from build123d import *

# Parameters (mm, degrees)
F1_DEPTH     = 2
F2_R         = 2
F3_R         = 2
F4_T4_DEPTH  = 22.7509646446
F4_T9_DEPTH  = 22.7509646446
F4_T14_DEPTH = 22.7509646446
F5_T4_DEPTH  = 22.7509646446
F5_T9_DEPTH  = 22.7509646446
F6_T4_DEPTH  = 22.7509646446


# Not quite as in the source:
# - a fillet or chamfer that OpenCascade refuses, or shapes differently, is made with other operations: its cross-section is extruded or revolved along the edge and cut away or added


with BuildPart() as f1:
    # F0 (on Top) → F1 (new body)
    with BuildSketch(Plane.XY):
        Polygon((-8.2, 10.65), (-14.2, 10.65), (-14.2, 0), (-8.2, -14.45), (-3.2, -14.45), (-3.2, -10.45), (-6.2, -10.45), (-6.2, -9.45), (-3.2, -9.45), (-3.2, -5.95), (-8.2, -5.95), (-8.2, 1), (-11.2, 1), (-11.2, 2), (-8.2, 2), (-8.2, 5.65), (-11.2, 5.65), (-11.2, 6.65), (-8.2, 6.65), align=None)
    extrude(amount=F1_DEPTH)

    # F2
    f2_edges = [f1.edges().sort_by_distance(p)[0] for p in [
        (-14.2, 10.65, 1),
        (-14.2, 0, 1),
        (-8.2, 10.65, 1),
        (-8.2, -14.45, 1),
        (-3.2, -14.45, 1),
        (-3.2, -5.95, 1),
    ]]
    fillet(f2_edges, radius=F2_R)

    # F3
    f3_edges = [f1.edges().sort_by_distance(p)[0] for p in [
        (-8.2, -5.95, 1),
    ]]
    fillet(f3_edges, radius=F3_R)

    # F4: chamfer of 1.5 x 4 on 3 edges, made by hand


with BuildPart() as f4_tool2:
    # F4_s3 → F4_t4 (new body)
    with BuildSketch(Plane.XY.offset(-10.3754823223)):
        Polygon((-12.2, 6.65), (-8.2, 8.15), (-8.2, 6.65), align=None)
    extrude(amount=F4_T4_DEPTH)

    split(bisect_by=Plane.YZ.offset(-11.2), keep=Keep.TOP)


with BuildPart() as f1_1:
    add(f1.part)

    # F4_t1: cut F4_tool2
    add(f4_tool2.part, mode=Mode.SUBTRACT)


with BuildPart() as f4_tool7:
    # F4_s8 → F4_t9 (new body)
    with BuildSketch(Plane.XY.offset(-10.3754823223)):
        Polygon((-12.2, 2), (-8.2, 3.5), (-8.2, 2), align=None)
    extrude(amount=F4_T9_DEPTH)

    split(bisect_by=Plane.YZ.offset(-11.2), keep=Keep.TOP)


with BuildPart() as f1_2:
    add(f1_1.part)

    # F4_t6: cut F4_tool7
    add(f4_tool7.part, mode=Mode.SUBTRACT)


with BuildPart() as f4_tool12:
    # F4_s13 → F4_t14 (new body)
    with BuildSketch(Plane.XY.offset(-10.3754823223)):
        Polygon((-3.2, -7.95), (-7.2, -9.45), (-3.2, -9.45), align=None)
    extrude(amount=F4_T14_DEPTH)

    split(bisect_by=Plane.YZ.offset(-6.2), keep=Keep.TOP)


with BuildPart() as f1_3:
    add(f1_2.part)

    # F4_t11: cut F4_tool12
    add(f4_tool12.part, mode=Mode.SUBTRACT)

    # F5: chamfer of 4 x 1.5 on 2 edges, made by hand


with BuildPart() as f5_tool2:
    # F5_s3 → F5_t4 (new body)
    with BuildSketch(Plane.XY.offset(-10.3754823223)):
        Polygon((-12.2, 5.65), (-8.2, 4.15), (-8.2, 5.65), align=None)
    extrude(amount=F5_T4_DEPTH)

    split(bisect_by=Plane.YZ.offset(-11.2), keep=Keep.TOP)


with BuildPart() as f1_4:
    add(f1_3.part)

    # F5_t1: cut F5_tool2
    add(f5_tool2.part, mode=Mode.SUBTRACT)


with BuildPart() as f5_tool7:
    # F5_s8 → F5_t9 (new body)
    with BuildSketch(Plane.XY.offset(-10.3754823223)):
        Polygon((-7.2, -10.45), (-3.2, -11.95), (-3.2, -10.45), align=None)
    extrude(amount=F5_T9_DEPTH)

    split(bisect_by=Plane.YZ.offset(-6.2), keep=Keep.TOP)


with BuildPart() as f1_5:
    add(f1_4.part)

    # F5_t6: cut F5_tool7
    add(f5_tool7.part, mode=Mode.SUBTRACT)

    # F6: chamfer of 4 x 1.5 on 1 edges, made by hand


with BuildPart() as f6_tool2:
    # F6_s3 → F6_t4 (new body)
    with BuildSketch(Plane.XY.offset(-10.3754823223)):
        Polygon((-12.2, 1), (-8.2, -0.5), (-8.2, 1), align=None)
    extrude(amount=F6_T4_DEPTH)

    split(bisect_by=Plane.YZ.offset(-11.2), keep=Keep.TOP)


with BuildPart() as f1_6:
    add(f1_5.part)

    # F6_t1: cut F6_tool2
    add(f6_tool2.part, mode=Mode.SUBTRACT)


solid = f1_6.part
Geometry: final body of the model. Coordinates: model frame, mm. A direction names the side the tool comes from. Coordinates: 2 decimals unless noted, no trailing zeros. Loops run counter-clockwise (first coordinate to the right, second up) from the corner with the lowest first, then second, coordinate; pieces in that order, holes last. Notation, with made-up numbers: (45.5, 75.5) - (70.5, 75.5) arc R21 cw to (70.5, 94.5) - close; hole circle Ø4 at (-37, 10.5). An arc over 180 degrees is marked (long way). Put each result on its own line as item: value. Start each with the question number.
Q1. Line query: line 1 (Y direction, x = -10.25, z = 1.75); line 2 (Y direction, x = -9, z = 1.45); line 3 (X direction, y = 8.5, z = 1.2). Output: solid intervals per line, ascending.
Q2. Cut plane C-C, the plane x = -3.75. Return loops of the section in (y, z).
Q3. Pin query (flat end, axial travel): pin 1 Ø1 at (y, z) = (-2.5, 0.5) entering from +X; pin 2 Ø0.9 at (y, z) = (6.5, 1.5) entering from +X; pin 3 Ø1.1 at (x, z) = (-5.5, 1) entering from +Y. Return the tip coordinate at first contact, or that it passes through.
Q4. Cut plane D-D, the plane y = 4.75. Return loops of the section in (x, z).
Q5. Set-up query: faces 5 (the cylindrical face through (-3.8, -13.88, 1.01)), 6 (the flat face through (-4.679, -8.505, 0.986)), 7 (the flat face through (-6, -5.95, 1)). Return all of +Z, -Z, +X, -X, +Y, -Y with unobstructed straight access to the full face (end or side cutting, diameter ignored); none if empty.
Q6. Cut plane B-B, the plane x = -9.75. Return loops of the section in (y, z).
Q7. Pull-direction query (Y, two-part tool) for faces 1 (the flat face through (-10, -2, 0)), 2 (the flat face through (-9.72, 0.07, 0.99)), 3 (the cylindrical face through (-13.6, 10.08, 1.01)), 4 (the cylindrical face through (-7.989, -14.104, 1.014)); classes: released by +Y, released by -Y, zero draft, split by the parting line, or undercut.
Q8. Cut plane A-A, the plane z = 0.5. Return loops of the section in (x, y) (3 decimals), and give its area (3 significant figures).
Filled sheet:
1. line 1: -9.51 to 0.27, 2.73 to 4.92, 7.38 to 10.65
1. line 2: -12.52 to -0.2, 3.2 to 4.45, 7.85 to 10.25
1. line 3: -14.2 to -8.2
2. outline: (-13.83, 0) - (-11.74, 0) - (-11.74, 2) - (-13.83, 2) - close; (-8.16, 0) - (-6.57, 0) - (-6.57, 2) - (-8.16, 2) - close
3. pin 1: x = -8.2
3. pin 2: x = -11.2
3. pin 3: y = -5.95
4. outline: (-14.2, 0) - (-9.8, 0) - (-9.8, 2) - (-14.2, 2) - close
5. face 5: +Z, -Z, +X, -Y
5. face 6: +Z, -Z, +X
5. face 7: +Z, -Z, +X, +Y
6. outline: (-10.72, 0) - (0.08, 0) - (0.08, 2) - (-10.72, 2) - close; (2.92, 0) - (4.73, 0) - (4.73, 2) - (2.92, 2) - close; (7.57, 0) - (10.6, 0) - (10.6, 2) - (7.57, 2) - close
7. face 1: zero draft
7. face 2: undercut
7. face 3: released by +Y
7. face 4: released by -Y
8. outline: (-14.2, 0.399) arc R2 ccw to (-14.047, -0.368) - (-8.712, -13.217) arc R2 ccw to (-6.865, -14.45) - (-5.2, -14.45) arc R2 ccw to (-3.2, -12.45) - (-3.2, -11.95) - (-6.2, -10.825) - (-6.2, -9.075) - (-3.2, -7.95) arc R2 ccw to (-5.2, -5.95) - (-6.2, -5.95) arc R2 cw to (-8.2, -3.95) - (-8.2, -0.5) - (-11.2, 0.625) - (-11.2, 2.375) - (-8.2, 3.5) - (-8.2, 4.15) - (-11.2, 5.275) - (-11.2, 7.025) - (-8.2, 8.15) - (-8.2, 8.65) arc R2 ccw to (-10.2, 10.65) - (-12.2, 10.65) arc R2 ccw to (-14.2, 8.65) - close
8. area: 121 mm²
